Design review of the part built by this model. Coordinates are the model's own, in mm. Give positions to 0.01 mm unless a question says otherwise; leave off trailing zeros. Loops run counter-clockwise (first coordinate to the right, second up) from the corner with the lowest first, then second, coordinate; pieces in that order, holes last.
from build123d import *

# Parameters (mm, degrees)
F2_R     = 2.54
F3_DEPTH = 76.2


with BuildPart() as f1:
    # F0 (on Front) → F1 (revolve)
    with BuildSketch(Plane.XZ):
        with BuildLine():
            Line((0, 3.81), (0, -3.81))
            ThreePointArc((0, -3.81), (3.81, 0), (0, 3.81))
        make_face()
    revolve(axis=Axis((0, 0, 0), (0, 0, -1)))

    # F2 (on Top) → F3 (join)
    with BuildSketch(Plane.XY):
        Circle(F2_R)
    extrude(amount=F3_DEPTH)

    # F4 (on face) → F5 (revolve)
    with BuildSketch(Plane.XY.offset(76.2)):
        with BuildLine():
            Line((0, -2.54), (0, -3.81))
            ThreePointArc((0, -3.81), (3.81, 0), (0, 3.81))
            Line((0, 3.81), (0, 2.54))
            ThreePointArc((0, 2.54), (1.7960512242, 1.7960512242), (2.54, 0))
            ThreePointArc((2.54, 0), (1.7960512242, -1.7960512242), (0, -2.54))
        make_face()
        with BuildLine():
            Line((0, 2.54), (0, -2.54))
            ThreePointArc((0, -2.54), (1.7960512242, -1.7960512242), (2.54, 0))
            ThreePointArc((2.54, 0), (1.7960512242, 1.7960512242), (0, 2.54))
        make_face()
    revolve(axis=Axis((0, 0, 76.2), (0, -1, 0)))


solid = f1.part
Q1. Take a section at A-A (z = 27.5). Give the boundary of the cut face in (x, y), plus the area to 3 significant figures.
Results:
outline: circle Ø5.08 at (0, 0)
area: 20.3 mm2
Q2. Insertion check: pin 1 (4 mm diameter, centred on x = 0.5, z = 71.5, fed in from +Y); pin 2 (1.5 mm diameter, centred on y = 0, z = 34, fed in from -X); pin 3 (3 mm diameter, centred on x = -2, z = 53.5, fed in from +Y). Each pin has a flat end and moves straight along its axis. Give the tip position at first contact, or say it passes through.
Results:
pin 1: stops at y = 2.66
pin 2: stops at x = -2.54
pin 3: stops at y = 2.49
Q3. Take a section at B-B (y = 0). Give the boundary of the cut face in (x, z), plus the area to 3 significant figures.
Results:
outline: (-2.54, 2.84) arc R3.81 ccw (long way) to (2.54, 2.84) - (2.54, 73.36) arc R3.81 ccw (long way) to (-2.54, 73.36) - close
area: 443 mm2
Q4. Wall thickness on line 1 (Z direction, x = 1, y = -2.75); line 2 (Y direction, x = 0, z = 70.5); line 3 (Z direction, x = -2.75, y = 0): over which ranges is each line inside the solid? List them lowest first.
Results:
line 1: z = -2.44 to 2.44, 73.76 to 78.64
line 2: y = -2.54 to 2.54
line 3: z = -2.64 to 2.64, 73.56 to 78.84
Q5. Take a section at C-C (x = 1.75). Give the boundary of the cut face in (y, z).
Results:
outline: (-1.84, 2.84) arc R3.38 ccw (long way) to (1.84, 2.84) - (1.84, 73.36) arc R3.38 ccw (long way) to (-1.84, 73.36) - close
